Input: part model. Units: mm. Frame: model coordinates. Face numbers are marked on the shaded views. Give positions to 0.01 mm unless a question says otherwise; leave off trailing zeros. Loops run counter-clockwise (first coordinate to the right, second up) from the corner with the lowest first, then second, coordinate; pieces in that order, holes last. Notation, with made-up numbers: M 24.25,-36.5 L 41.25,-36.5 A10 ccw 41.25,-18.5 Z; hole C 54.5,84.5 d6. An arc over 180 degrees is marked long. Use CSV: the item, a comma, the result in double quotes. Start each with the question number.
from build123d import *

# Parameters (mm, degrees)
SKETCH1_R           = 159.375
BOSS_EXTRUDE2_DEPTH = 60
BOSS_EXTRUDE4_DEPTH = 1


with BuildPart() as part:
    # Sketch1 → Boss-Extrude2 (new body)
    with BuildSketch(Plane(origin=(0, 0, 0), x_dir=(1, 0, 0), z_dir=(0, 1, 0))):
        with Locations(Location((0, 0, 0), (0, 0, 270))):
            Circle(SKETCH1_R)
    extrude(amount=BOSS_EXTRUDE2_DEPTH)

    # Sketch3 → Boss-Extrude4 (add)
    with BuildSketch(Plane(origin=(0, 60, 0), x_dir=(1, 0, 0), z_dir=(0, 1, 0))):
        Polygon((63.75, 9.990395), (63.75, 0), (63.75, -9.990395), (64.75, -9.990395), (64.75, 9.990395), align=None)
    extrude(amount=BOSS_EXTRUDE4_DEPTH)


solid = part.part
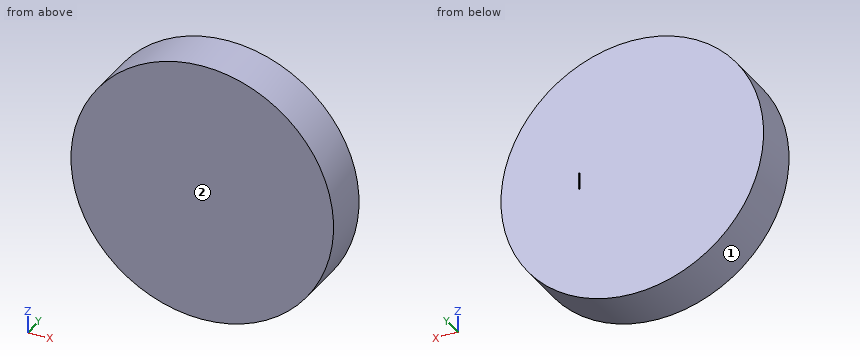
Item 1: First-contact query: pin 1 Ø12 at (y, z) = (13.5, 89) entering from -X; pin 2 Ø2 at (y, z) = (50.5, 121) entering from -X; pin 3 Ø2 at (x, y) = (48.5, 21) entering from -Z. Flat tips, straight axial feed; report the tip coordinate or a pass-through.
Item 2: Material intervals for line 1 (Z direction, x = 4, y = 21); line 2 (Y direction, x = -51.5, z = -40); line 3 (Z direction, x = 1.5, y = 41.5), sorted ascending.
Item 3: Section C-C (y = 29). Output: boundary loops of the cut face in (x, z) (3 decimals), then the cut area to 3 significant figures.
Item 4: Mould query, pull axis X, two halves, no side actions, for the marked faces 1 and 2. Classes: +X half, -X half, draft (parallel to the pull), parting line (faces both ways), or undercut.
Item 5: Section D-D (x = -98). Output: boundary loops of the cut face in (y, z).
Item 6: Section A-A (z = 0). Output: boundary loops of the cut face in (x, y) (3 decimals), then the cut area to 3 significant figures.
Item 7: Section B-B (x = 0). Output: boundary loops of the cut face in (y, z) (3 decimals), then the cut area to 3 significant figures.
Recorded:
1,pin 1,"x = -136.06"
1,pin 2,"x = -104.88"
1,pin 3,"z = -152.13"
2,line 1,"-159.32 to 159.32"
2,line 2,"0 to 60"
2,line 3,"-159.37 to 159.37"
3,outline,"C 0,0 d318.75"
3,area,"79,800 mm²"
4,face 1,"parting line"
4,face 2,"draft"
5,outline,"M 0,-125.68 L 60,-125.68 L 60,125.68 L 0,125.68 Z"
6,outline,"M -159.375,0 L 159.375,0 L 159.375,60 L 64.75,60 L 64.75,61 L 63.75,61 L 63.75,60 L -159.375,60 Z"
6,area,"19,100 mm²"
7,outline,"M 0,-159.375 L 60,-159.375 L 60,159.375 L 0,159.375 Z"
7,area,"19,100 mm²"
